Geometry: see drawing. Coordinates: mm, zero at the bounding-box minimum. A direction names the side the tool comes from. Coordinates: 2 decimals unless noted, no trailing zeros. Write each loop counter-clockwise with the first axis right and the second up, starting at its lowest first coordinate (ties: lowest second). Pieces come first, ordered by that corner, then holes. Notation, with made-up numbers: (67, 62.5) - (110, 62.5) arc R19 cw to (110, 98.5) - close; hole circle Ø3 at (27.5, 4.5). An arc over 180 degrees is marked (long way). Use a Markdown table: item, result. Add a question column.
Q1. Set-up query: the marked faces 1 and 2. Return all of +Z, -Z, +X, -X, +Y, -Y with unobstructed straight access to the full face (end or side cutting, diameter ignored); none if empty.
Q2. Pin query (flat end, axial travel): P1, Ø3.5, axis at x = 7.5, z = 3, coming from the -Y side. Return the tip coordinate at first contact, or that it passes through.
Q3. Section query A-A (z = 2). Return the cut outline in (x, y), then the cut area to 3 significant figures.
Q4. Section query D-D (y = 22.25). Return the cut outline in (x, z).
Q5. Mould query, pull axis Z, two halves, no side actions, for the marked faces 3, 4 and 5. Classes: released by +Z, released by -Z, zero draft, split by the parting line, or undercut.
Q6. Section query B-B (y = 13). Return the cut outline in (x, z).
Q7. Material intervals for probe 1 along Z at (x, y) = (19.5, 16.5); probe 2 along Z at (x, y) = (16.25, 3.5); probe 3 along Y at (x, z) = (12, 4), sorted ascending. Write a range as from..to.
Q8. Section query C-C (x = 4.25). Return the cut outline in (y, z).
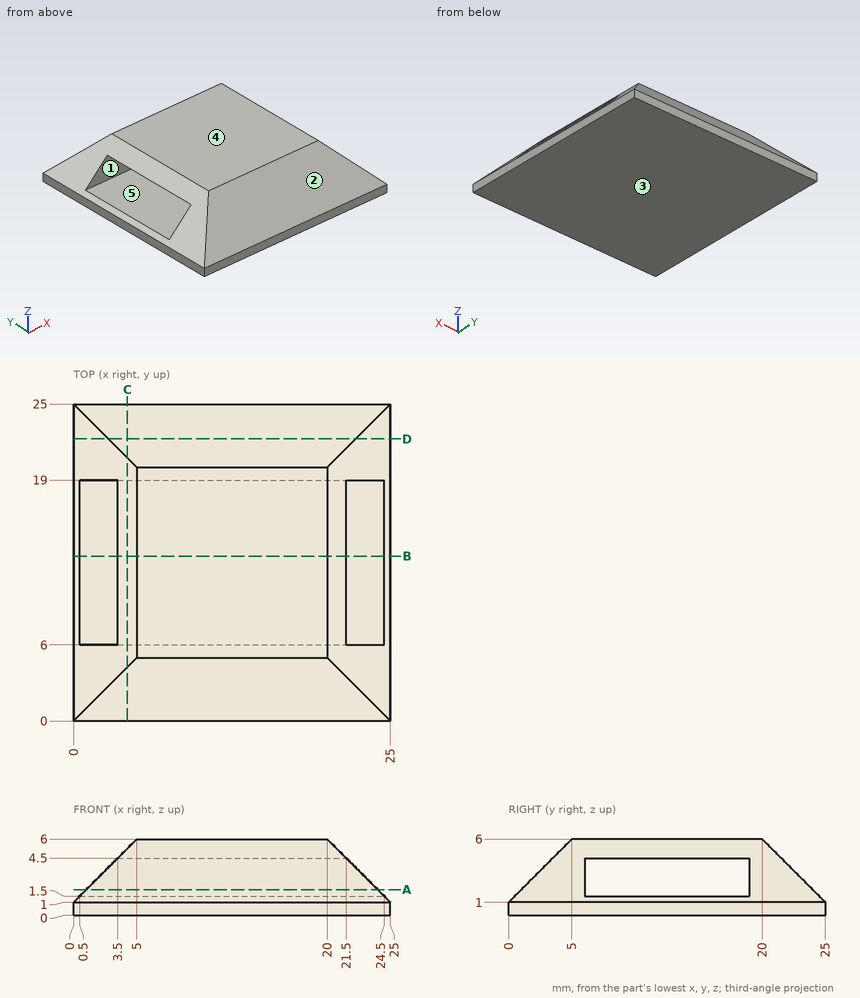
Values follow:
| question | item | result |
|---|---|---|
| 1 | face 1 | +X, -X |
| 1 | face 2 | +Z, +X, -X, -Y |
| 2 | P1 | y = 0.25 |
| 3 | outline | (1, 1) - (24, 1) - (24, 6) - (1, 6) - close; (1, 19) - (24, 19) - (24, 24) - (1, 24) - close |
| 3 | area | 230 mm2 |
| 4 | outline | (0, 0) - (25, 0) - (25, 1) - (22.25, 3.75) - (2.75, 3.75) - (0, 1) - close |
| 5 | face 3 | released by -Z |
| 5 | face 4 | released by +Z |
| 5 | face 5 | undercut |
| 6 | outline | (0, 0) - (25, 0) - (25, 1) - (24.5, 1.5) - (0.5, 1.5) - (0, 1) - close; (3.5, 4.5) - (21.5, 4.5) - (20, 6) - (5, 6) - close |
| 7 | probe 1 | 0..1.5, 4.5..6 |
| 7 | probe 2 | 0..4.5 |
| 7 | probe 3 | 3..6, 19..22 |
| 8 | outline | (0, 0) - (25, 0) - (25, 1) - (20.75, 5.25) - (4.25, 5.25) - (0, 1) - close; hole (6, 1.5) - (19, 1.5) - (19, 4.5) - (6, 4.5) - close |
